from build123d import *

# Parameters (mm, degrees)
SKETCH3_R           = 15.9131
SKETCH3_R_2         = 12.7254
BOSS_EXTRUDE1_DEPTH = 19.05
SKETCH4_R           = 19.05
SKETCH4_R_2         = 15.9131
BOSS_EXTRUDE2_DEPTH = 4.7625
CHAMFER1_SIZE       = 0.254508
FILLET1_R           = 0.2227834


with BuildPart() as part:
    # Sketch3 → Boss-Extrude1 (new body)
    with BuildSketch(Plane.XY):
        with Locations(Location((0, 0, 0), (0, 0, 180))):
            Circle(SKETCH3_R)
        with Locations(Location((0, 0, 0), (0, 0, 180))):
            Circle(SKETCH3_R_2, mode=Mode.SUBTRACT)
    extrude(amount=BOSS_EXTRUDE1_DEPTH)

    # Sketch4 → Boss-Extrude2 (add)
    with BuildSketch(Plane.XY):
        with Locations(Location((0, 0, 0), (0, 0, 180))):
            Circle(SKETCH4_R)
        with Locations(Location((0, 0, 0), (0, 0, 180))):
            Circle(SKETCH4_R_2, mode=Mode.SUBTRACT)
    extrude(amount=BOSS_EXTRUDE2_DEPTH)

    # Chamfer1
    chamfer1_edges = [part.edges().sort_by_distance(p)[0] for p in [
        (12.7254, 0, 0),
        (12.7254, 0, 19.05),
    ]]
    chamfer(chamfer1_edges, length=CHAMFER1_SIZE)

    # Fillet1
    fillet1_edges = [part.edges().sort_by_distance(p)[0] for p in [
        (19.05, 0, 4.7625),
        (19.05, 0, 0),
        (15.9131, 0, 4.7625),
        (15.9131, 0, 19.05),
    ]]
    fillet(fillet1_edges, radius=FILLET1_R)


solid = part.part
Geometry: final body of the model. Coordinates: model frame, mm. Give positions to 0.01 mm unless a question says otherwise; leave off trailing zeros. Loops run counter-clockwise (first coordinate to the right, second up) from the corner with the lowest first, then second, coordinate; pieces in that order, holes last. Notation, with made-up numbers: M -1,81.25 L 20,81.25 A25 ccw 20,97.25 Z; hole C 33.5,71.25 d10. An arc over 180 degrees is marked long. Put each result on its own line as item: value. Start each with the question number.
1) Ray query, line 1 along Y through (x, z) = (0.5, 17); line 2 along X through (y, z) = (-1, 11); line 3 along X through (y, z) = (10, 15). Return the intervals inside material, ascending.
2) Cut plane D-D (z = 2.5). Output: boundary loops of the cut face in (x, y).
3) Cut plane C-C (z = 5.75). Output: boundary loops of the cut face in (x, y), then the cut area to 3 significant figures.
4) Contact query for flat-ended pins moving along their axis: pin 1 (5 mm diameter, centred on y = -5, z = 10, fed in from +X); pin 2 (1 mm diameter, centred on y = -4, z = 9.5, fed in from +X); pin 3 (10 mm diameter, centred on x = 1.5, y = -7.5, fed in from -Z); pin 4 (6 mm diameter, centred on x = 1.5, z = 9.5, fed in from +Y). Output: stop coordinate, or through.
5) Cut plane A-A (y = 0). Output: boundary loops of the cut face in (x, z).
6) Pull-direction query (Y, two-part tool) for faces 1 (the flat face through (-13.9, -8.5, 4.762)), 2 (the cylindrical face through (12.63, 9.68, 11.81)), 3 (the cylindrical face through (1.657, -12.617, 9.395)); classes: pulls with the +Y half, pulls with the -Y half, needs draft (parallel to the pull), parting line crosses it, or undercut.
Verdict:
1. line 1: -15.91 to -12.72, 12.72 to 15.91
1. line 2: -15.88 to -12.69, 12.69 to 15.88
1. line 3: -12.38 to -7.87, 7.87 to 12.38
2. outline: C 0,0 d38.1; hole C 0,0 d25.45
3. outline: C 0,0 d31.83; hole C 0,0 d25.45
3. area: 287 mm2
4. pin 1: x = 15.72
4. pin 2: x = 15.52
4. pin 3: through
4. pin 4: y = 15.91
5. outline: M -19.05,0.22 A0.22 ccw -18.83,0 L -12.98,0 L -12.73,0.25 L -12.73,18.8 L -12.98,19.05 L -15.69,19.05 A0.22 ccw -15.91,18.83 L -15.91,4.99 A0.22 cw -16.14,4.76 L -18.83,4.76 A0.22 ccw -19.05,4.54 Z; M 12.73,0.25 L 12.98,0 L 18.83,0 A0.22 ccw 19.05,0.22 L 19.05,4.54 A0.22 ccw 18.83,4.76 L 16.14,4.76 A0.22 cw 15.91,4.99 L 15.91,18.83 A0.22 ccw 15.69,19.05 L 12.98,19.05 L 12.73,18.8 Z
6. face 1: needs draft
6. face 2: parting line crosses it
6. face 3: undercut
